```python
from build123d import *

# Parameters (mm, degrees)
SKETCH_1_R      = 17
SKETCH_1_R_2    = 1.65
EXTRUDE_1_DEPTH = 3


with BuildPart() as part:
    # 草图1 → 凸台-拉伸1 (new body)
    with BuildSketch(Plane.XY):
        Circle(SKETCH_1_R)
        with BuildLine():
            ThreePointArc((2.2, -13), (0, -15.2), (-2.2, -13))
            Line((-2.2, -13), (-2.2, -12))
            ThreePointArc((-2.2, -12), (0, -9.8), (2.2, -12))
            Line((2.2, -12), (2.2, -13))
        make_face(mode=Mode.SUBTRACT)
        with Locations((0, -7)):
            Circle(SKETCH_1_R_2, mode=Mode.SUBTRACT)
        with BuildLine():
            ThreePointArc((-13, -2.2), (-15.2, 0), (-13, 2.2))
            Line((-13, 2.2), (-12, 2.2))
            ThreePointArc((-12, 2.2), (-10.444365081, 1.555634919), (-9.8, 0))
            ThreePointArc((-9.8, 0), (-10.444365081, -1.555634919), (-12, -2.2))
            Line((-12, -2.2), (-13, -2.2))
        make_face(mode=Mode.SUBTRACT)
        with Locations((-7, 0)):
            Circle(SKETCH_1_R_2, mode=Mode.SUBTRACT)
        Circle(SKETCH_1_R_2, mode=Mode.SUBTRACT)
        with Locations((7, 0)):
            Circle(SKETCH_1_R_2, mode=Mode.SUBTRACT)
        with Locations((0, 7)):
            Circle(SKETCH_1_R_2, mode=Mode.SUBTRACT)
        with BuildLine():
            Line((13, -2.2), (12, -2.2))
            ThreePointArc((12, -2.2), (9.8, 0), (12, 2.2))
            Line((12, 2.2), (13, 2.2))
            ThreePointArc((13, 2.2), (14.555634919, 1.555634919), (15.2, 0))
            ThreePointArc((15.2, 0), (14.555634919, -1.555634919), (13, -2.2))
        make_face(mode=Mode.SUBTRACT)
        with BuildLine():
            Line((-2.2, 12), (-2.2, 13))
            ThreePointArc((-2.2, 13), (0, 15.2), (2.2, 13))
            Line((2.2, 13), (2.2, 12))
            ThreePointArc((2.2, 12), (0, 9.8), (-2.2, 12))
        make_face(mode=Mode.SUBTRACT)
    extrude(amount=EXTRUDE_1_DEPTH)


solid = part.part
```
Design review of the part built by this model. Coordinates are the model's own, in mm. Give positions to 0.01 mm unless a question says otherwise; leave off trailing zeros. Write each loop counter-clockwise with the first axis right and the second up, starting at its lowest first coordinate (ties: lowest second). Pieces come first, ordered by that corner, then holes. Notation, with made-up numbers: (-37, -9.75) -> (-33, -9.75) arc R30 ccw to (-33, 12.25) -> close; hole circle Ø5 at (67.25, 2.5). An arc over 180 degrees is marked (long way). Answer in a Markdown table with one row per item.
(1) To check wall thickness, follow probe 1 along Y at (x, z) = (0, 1.4); probe 2 along Y at (x, z) = (-0.5, 1.85); probe 3 along X at (y, z) = (1.5, 1.9). State the ranges of each line that lie inside material, in increasing order.
Results:
| item | result |
|---|---|
| probe 1 | -17 to -15.2, -9.8 to -8.65, -5.35 to -1.65, 1.65 to 5.35, 8.65 to 9.8, 15.2 to 17 |
| probe 2 | -16.99 to -15.14, -9.86 to -8.57, -5.43 to -1.57, 1.57 to 5.43, 8.57 to 9.86, 15.14 to 16.99 |
| probe 3 | -16.93 to -14.61, -10.39 to -7.69, -6.31 to -0.69, 0.69 to 6.31, 7.69 to 10.39, 14.61 to 16.93 |
(2) Consider section B-B (z = 1.85). Count the separate pieces of the cut face and the enclosed holes in it, then the cut area to 3 significant figures.
Results:
| item | result |
|---|---|
| separate pieces | 1 |
| enclosed holes | 9 |
| area | 787 mm2 |
(3) Mouldability with a two-part tool opening along X and no side actions: class faces 1 (the cylindrical face through (9.139, 14.334, 1.479)), 2 (the flat face through (-2.2, 12.5, 1.5)) as +X half, -X half, draft (parallel to the pull), parting line (faces both ways), or undercut.
Results:
| item | result |
|---|---|
| face 1 | parting line |
| face 2 | undercut |
(4) Consider section C-C (y = -6). State the section outline as (x, z) points.
Results:
| item | result |
|---|---|
| outline | (-15.91, 0) -> (-1.31, 0) -> (-1.31, 3) -> (-15.91, 3) -> close; (1.31, 0) -> (15.91, 0) -> (15.91, 3) -> (1.31, 3) -> close |
(5) Consider section D-D (x = -7). State the section outline as (y, z) points, then the cut area to 3 significant figures.
Results:
| item | result |
|---|---|
| outline | (-15.49, 0) -> (-1.65, 0) -> (-1.65, 3) -> (-15.49, 3) -> close; (1.65, 0) -> (15.49, 0) -> (15.49, 3) -> (1.65, 3) -> close |
| area | 83.1 mm2 |
(6) Consider section A-A (x = 0). State the section outline as (y, z) points.
Results:
| item | result |
|---|---|
| outline | (-17, 0) -> (-15.2, 0) -> (-15.2, 3) -> (-17, 3) -> close; (-9.8, 0) -> (-8.65, 0) -> (-8.65, 3) -> (-9.8, 3) -> close; (-5.35, 0) -> (-1.65, 0) -> (-1.65, 3) -> (-5.35, 3) -> close; (1.65, 0) -> (5.35, 0) -> (5.35, 3) -> (1.65, 3) -> close; (8.65, 0) -> (9.8, 0) -> (9.8, 3) -> (8.65, 3) -> close; (15.2, 0) -> (17, 0) -> (17, 3) -> (15.2, 3) -> close |
(7) Clearance check with flat-ended pins moving along their axes: pin 1 (0.5 mm diameter, centred on x = -12.5, z = 1, fed in from +Y); pin 2 (0.8 mm diameter, centred on y = 12.5, z = 2, fed in from -X); pin 3 (1.5 mm diameter, centred on y = -6, z = 2.5, fed in from +X). State where each tip first meets the part, or that it passes through.
Results:
| item | result |
|---|---|
| pin 1 | y = 11.79 |
| pin 2 | x = -11.94 |
| pin 3 | x = 16.17 |
